Answer from the drawing. Dimensions are ordinates in mm from the lowest x, y and z of the part. A direction names the side the tool comes from. Round coordinates to 2 decimals unless told otherwise and drop trailing zeros. Write each loop counter-clockwise with the first axis right and the second up, starting at its lowest first coordinate (ties: lowest second). Pieces come first, ordered by that corner, then holes.
1. Find section C-C (x = 101.6). Write down the section's boundary in (y, z), and give its area (3 significant figures).
2. Find section A-A (z = 30). Write down the section's boundary in (x, y), and give its area (3 significant figures).
3. Find section D-D (z = 101.6). Write down the section's boundary in (x, y), and give its area (3 significant figures).
4. Flat-ended cylindrical pins translate along their axes: pin 1 Ø2 at (x, y) = (76.5, 99.5) entering from -Z; pin 2 Ø1 at (y, z) = (88, 71.5) entering from -X; pin 3 Ø1 at (x, z) = (79, 25) entering from +Y. Find the tip coordinate at first contact, or state that the pin passes through.
5. Determine the mould class of the marked faces 1, 2, 3 and 4 for opening direction Y: pulls with the +Y half, pulls with the -Y half, needs draft (parallel to the pull), parting line crosses it, or undercut.
6. Find section B-B (x = 180.5). Write down the section's boundary in (y, z).
7. A tool of negligible diameter and unlimited length cuts with its end or side. For the marked faces 5, 6 and 7, from which of +Z, -Z, +X, -X, +Y, -Y can it reach the whole face along a straight path? Write none if from no direction.
8. Straight lines are drawn through the part: probe 1 along Y at (x, z) = (38.5, 137.5); probe 2 along Z at (x, y) = (102.5, 73.5). For each, find the intervals that lie inside material, in ascending order.
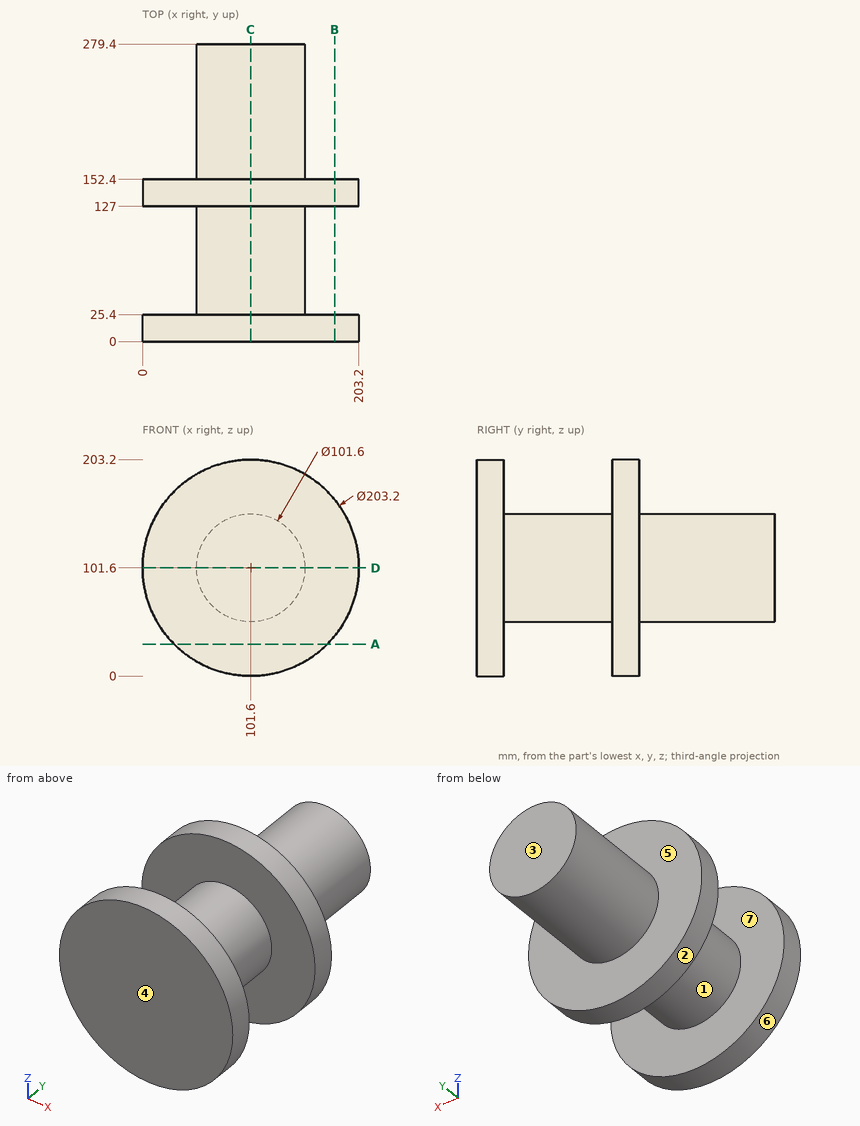
Worked answers:
1. outline: (0, 0) - (25.4, 0) - (25.4, 50.8) - (127, 50.8) - (127, 0) - (152.4, 0) - (152.4, 50.8) - (279.4, 50.8) - (279.4, 152.4) - (152.4, 152.4) - (152.4, 203.2) - (127, 203.2) - (127, 152.4) - (25.4, 152.4) - (25.4, 203.2) - (0, 203.2) - close
1. area: 33,500 mm2
2. outline: (29.52, 0) - (173.68, 0) - (173.68, 25.4) - (29.52, 25.4) - close; (29.52, 127) - (173.68, 127) - (173.68, 152.4) - (29.52, 152.4) - close
2. area: 7,320 mm2
3. outline: (0, 0) - (203.2, 0) - (203.2, 25.4) - (152.4, 25.4) - (152.4, 127) - (203.2, 127) - (203.2, 152.4) - (152.4, 152.4) - (152.4, 279.4) - (50.8, 279.4) - (50.8, 152.4) - (0, 152.4) - (0, 127) - (50.8, 127) - (50.8, 25.4) - (0, 25.4) - close
3. area: 33,500 mm2
4. pin 1: stops at z = 56.88
4. pin 2: stops at x = 60.31
4. pin 3: stops at y = 152.4
5. face 1: undercut
5. face 2: needs draft
5. face 3: pulls with the +Y half
5. face 4: pulls with the -Y half
6. outline: (0, 37.59) - (25.4, 37.59) - (25.4, 165.61) - (0, 165.61) - close; (127, 37.59) - (152.4, 37.59) - (152.4, 165.61) - (127, 165.61) - close
7. face 5: +Y
7. face 6: +Y, -Y
7. face 7: none
8. probe 1: y = 0 to 25.4, 127 to 152.4
8. probe 2: z = 50.81 to 152.39
